Work out the finished part from the listing and answer in its coordinate system (mm). A direction names the side the tool comes from. Give positions to 0.01 mm unless a question says otherwise; leave off trailing zeros. Loops run counter-clockwise (first coordinate to the right, second up) from the corner with the lowest first, then second, coordinate; pieces in that order, holes last. Notation, with made-up numbers: (59.5, 42.5) - (115.5, 42.5) arc R22 ccw to (115.5, 62.5) - close; hole circle Ø11 at (-15.75, 32.5). An arc over 180 degrees is marked (long way). Use CSV: the item, a comma, the result in double quotes.
from build123d import *

# Parameters (mm, degrees)
SKETCH1_W           = 19
SKETCH1_H           = 3
BOSS_EXTRUDE1_DEPTH = 3


with BuildPart() as part:
    # Sketch1 → Boss-Extrude1 (new body)
    with BuildSketch(Plane.XY):
        Polygon((0, 0), (0, 30), (18, 30), (18, 27), (37, 27), (37, 30), (55, 30), (55, 0), (48, 0), (48, -3), (38, -3), (38, 0), (31, 0), (24, 0), (17, 0), (17, -3), (7, -3), (7, 0), align=None)
        with Locations((27.5, 5.5)):
            Rectangle(SKETCH1_W, SKETCH1_H, mode=Mode.SUBTRACT)
    extrude(amount=BOSS_EXTRUDE1_DEPTH)


solid = part.part
Item 1: A cutting plane is placed at A-A on y = 6. Determine the outline of the cut face in (x, z), and give its area (3 significant figures).
Determined:
outline,"(0, 0) - (18, 0) - (18, 3) - (0, 3) - close; (37, 0) - (55, 0) - (55, 3) - (37, 3) - close"
area,"108 mm²"
Item 2: A cutting plane is placed at C-C on z = 2.45. Determine the outline of the cut face in (x, y), and give its area (3 significant figures).
Determined:
outline,"(0, 0) - (7, 0) - (7, -3) - (17, -3) - (17, 0) - (38, 0) - (38, -3) - (48, -3) - (48, 0) - (55, 0) - (55, 30) - (37, 30) - (37, 27) - (18, 27) - (18, 30) - (0, 30) - close; hole (18, 4) - (37, 4) - (37, 7) - (18, 7) - close"
area,"1,600 mm²"
Item 3: A cutting plane is placed at B-B on x = 19. Determine the outline of the cut face in (y, z).
Determined:
outline,"(0, 0) - (4, 0) - (4, 3) - (0, 3) - close; (7, 0) - (27, 0) - (27, 3) - (7, 3) - close"
Item 4: Find the intervals of material crossed by line 1 (Y direction, x = 30, z = 0.2); line 2 (X direction, y = -0.5, z = 2.1); line 3 (X direction, y = 6.5, z = 0.85), in increasing order.
Determined:
line 1,"y = 0 to 4, 7 to 27"
line 2,"x = 7 to 17, 38 to 48"
line 3,"x = 0 to 18, 37 to 55"
Item 5: For faces 4 (the flat face through (27, 7, 1)), 5 (the flat face through (52, 0, 1)), 6 (the flat face through (27, 0, 1)), determine the directions among +Z, -Z, +X, -X, +Y, -Y from which every point of the face is accessible in a straight line to the end or side of a thin tool.
Determined:
face 4,"+Z, -Z"
face 5,"+Z, -Z, +X, -Y"
face 6,"+Z, -Z, -Y"
Item 6: The mould has two halves that part along X. Classify faces 1 (the flat face through (12, -3, 1)), 2 (the flat face through (38, -2, 1)), 3 (the flat face through (7, -2, 1)): pulls with the +X half, pulls with the -X half, needs draft (parallel to the pull), parting line crosses it, or undercut.
Determined:
face 1,"needs draft"
face 2,"undercut"
face 3,"pulls with the -X half"
Item 7: Given P1, Ø0.9, axis at x = 50.5, z = 1, coming from the -Y side; P2, Ø1.5, axis at x = 27, z = 1, coming from the +Y side; P3, Ø1.5, axis at y = -1, z = 1, coming from the -X side, each flat-ended and moving along its own axis, determine where each tip first touches the part or whether it passes through.
Determined:
P1,"stops at y = 0"
P2,"stops at y = 27"
P3,"stops at x = 7"
